from build123d import *

# Parameters (mm, degrees)
SKETCH1_W           = 29.8
SKETCH1_H           = 27
BOSS_EXTRUDE1_DEPTH = 1
BOSS_EXTRUDE2_DEPTH = 2.4
SKETCH3_W           = 31.8
SKETCH3_H           = 3
BOSS_EXTRUDE3_DEPTH = 1
SKETCH5_W           = 1
SKETCH5_H           = 25
BOSS_EXTRUDE4_DEPTH = 1
SKETCH6_W           = 1
SKETCH6_H           = 25
BOSS_EXTRUDE5_DEPTH = 1


with BuildPart() as part:
    # Sketch1 → Boss-Extrude1 (new body)
    with BuildSketch(Plane(origin=(0, 0, 0), x_dir=(1, 0, 0), z_dir=(0, 1, 0))):
        Rectangle(SKETCH1_W, SKETCH1_H)
    extrude(amount=BOSS_EXTRUDE1_DEPTH)

    # Sketch2 → Boss-Extrude2 (add)
    with BuildSketch(Plane.XZ):
        Polygon((15.9, -13.5), (15.9, 14.5), (-15.9, 14.5), (-15.9, -13.5), (-14.9, -13.5), (-14.9, 13.5), (14.9, 13.5), (14.9, -13.5), align=None)
    extrude(amount=-BOSS_EXTRUDE2_DEPTH)

    # Sketch3 → Boss-Extrude3 (add)
    with BuildSketch(Plane(origin=(0, 2.4, 0), x_dir=(1, 0, 0), z_dir=(0, 1, 0))):
        with Locations((0, -13)):
            Rectangle(SKETCH3_W, SKETCH3_H)
    extrude(amount=BOSS_EXTRUDE3_DEPTH)

    # Sketch5 → Boss-Extrude4 (add)
    with BuildSketch(Plane(origin=(0, 2.4, 0), x_dir=(1, 0, 0), z_dir=(0, 1, 0))):
        with Locations((15.4, 1)):
            Rectangle(SKETCH5_W, SKETCH5_H)
    extrude(amount=BOSS_EXTRUDE4_DEPTH)

    # Sketch6 → Boss-Extrude5 (add)
    with BuildSketch(Plane(origin=(0, 2.4, 0), x_dir=(1, 0, 0), z_dir=(0, 1, 0))):
        with Locations((-15.4, 1)):
            Rectangle(SKETCH6_W, SKETCH6_H)
    extrude(amount=BOSS_EXTRUDE5_DEPTH)


solid = part.part
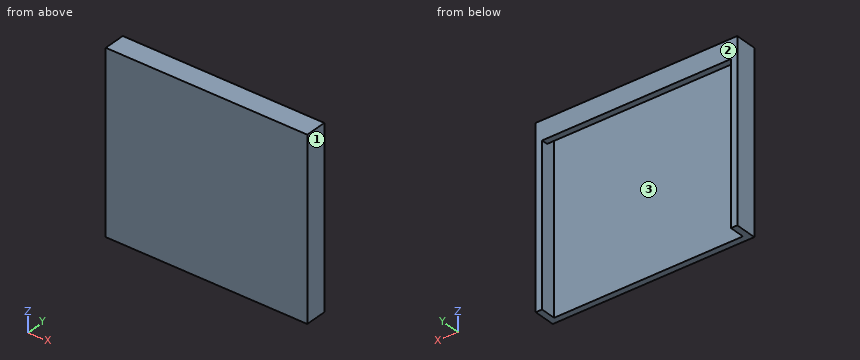
Read the model definition and answer for the solid it produces. Units are mm, in the model's axes. Face numbers are marked on the shaded views. Coordinates: 2 decimals unless noted, no trailing zeros. Order: outer loops, then holes, each group sorted by start corner. A loop starts at its lowest first (then second) coordinate and runs counter-clockwise, first axis right, second up. Notation, with made-up numbers: M -17,66.25 L 20,66.25 A18 cw 20,78.25 Z; hole C -5.75,-19 d6. An arc over 180 degrees is marked long. Put each result on its own line as item: value. Start each with the question number.
Item 1: Section A-A, the plane y = 2 is taken. Determine the outline of the cut face in (x, z).
Item 2: The mould has two halves that part along X. Classify the marked faces 1, 2 and 3: +X half, -X half, draft (parallel to the pull), parting line (faces both ways), or undercut.
Item 3: Given pin 1 Ø2 at (x, z) = (6.5, 1) entering from +Y; pin 2 Ø5 at (x, z) = (9.5, -1.5) entering from -Y; pin 3 Ø1.1 at (x, y) = (0, 3) entering from -Z, each flat-ended and moving along its own axis, determine where each tip first touches the part or whether it passes through.
Item 4: Section C-C, the plane z = 12.5 is taken. Determine the outline of the cut face in (x, y), plus the area to 3 significant figures.
Item 5: Consider probe 1 along X at (y, z) = (2.05, -11.5); probe 2 along Y at (x, z) = (-13, -5.5); probe 3 along Z at (x, y) = (10.5, 2.6). Determine where each line is inside the solid, lowest interval first. Write a range as [from, to].
Item 6: Section B-B, the plane z = 7 is taken. Determine the outline of the cut face in (x, y), plus the area to 3 significant figures.
Computed:
1. outline: M -15.9,-13.5 L -14.9,-13.5 L -14.9,13.5 L 14.9,13.5 L 14.9,-13.5 L 15.9,-13.5 L 15.9,14.5 L -15.9,14.5 Z
2. face 1: +X half
2. face 2: draft
2. face 3: undercut
3. pin 1: stops at y = 1
3. pin 2: stops at y = 0
3. pin 3: stops at z = 11.5
4. outline: M -15.9,0 L 15.9,0 L 15.9,3.4 L -15.9,3.4 Z; hole M -14.9,1 L 14.9,1 L 14.9,2.4 L -14.9,2.4 Z
4. area: 66.4 mm2
5. probe 1: x = [-15.9, -14.9], [14.9, 15.9]
5. probe 2: y = [0, 1]
5. probe 3: z = [11.5, 14.5]
6. outline: M -15.9,0 L 15.9,0 L 15.9,3.4 L 14.9,3.4 L 14.9,1 L -14.9,1 L -14.9,3.4 L -15.9,3.4 Z
6. area: 36.6 mm2
